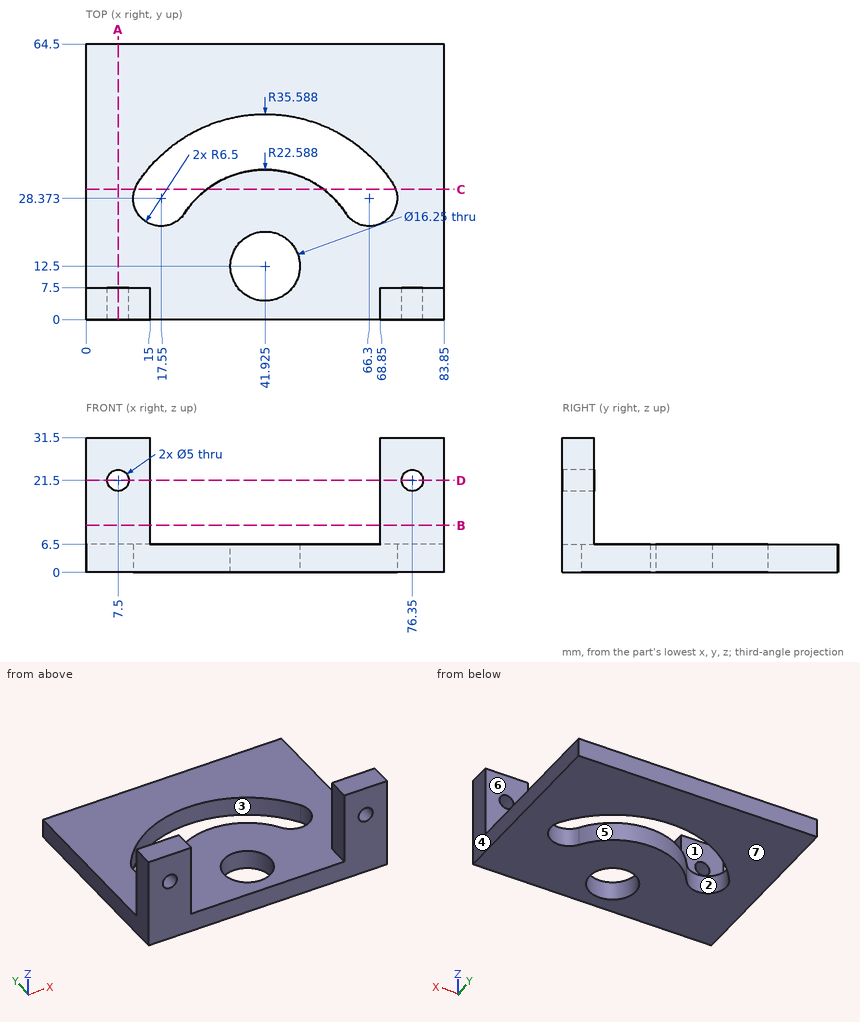
Source: three-view drawing plus pictorial views. Frame: mm from the lowest corner of the part. A direction names the side the tool comes from. Give positions to 0.01 mm unless a question says otherwise; leave off trailing zeros. Order: outer loops, then holes, each group sorted by start corner. A loop starts at its lowest first (then second) coordinate and runs counter-clockwise, first axis right, second up. Notation, with made-up numbers: (-15, 54.5) -> (30, 54.5) arc R24 ccw to (30, 86.5) -> close; hole circle Ø10 at (-4.75, 21). An arc over 180 degrees is marked (long way). Put each result on its own line as item: value.
Q1. Material intervals for L1, parallel to X at y = 4, z = 21; L2, parallel to Y at x = 21, z = 1.5 (1 decimal); L3, parallel to Z at x = 65, y = 46, sorted ascending.
Here are the results:
L1: x = 0 to 5.05, 9.95 to 15, 68.85 to 73.9, 78.8 to 83.85
L2: y = 0 to 22.9, 41.3 to 64.5
L3: z = 0 to 6.5
Q2. Section C-C, the plane y = 30.5. Return loops of the section in (x, z), then the cut area to 3 significant figures.
Here are the results:
outline: (0, 0) -> (11.41, 0) -> (11.41, 6.5) -> (0, 6.5) -> close; (28.28, 0) -> (55.57, 0) -> (55.57, 6.5) -> (28.28, 6.5) -> close; (72.44, 0) -> (83.85, 0) -> (83.85, 6.5) -> (72.44, 6.5) -> close
area: 326 mm^2
Q3. Reachability of the marked faces 5, 6 and 7 from +Z, -Z, +X, -X, +Y, -Y: full face, straight path, thin tool, end or side. Return the list, or none.
Here are the results:
face 5: +Z, -Z
face 6: +Z, +X, -X, +Y
face 7: -Z, +X, -X, +Y, -Y
Q4. Pin query (flat end, axial travel): pin 1 (12 mm diameter, centred on x = 75.5, z = 16.5, fed in from +Y); pin 2 (2 mm diameter, centred on x = 22, y = 55, fed in from +Z). Return the tip coordinate at first contact, or that it passes through.
Here are the results:
pin 1: stops at y = 7.5
pin 2: stops at z = 6.5
Q5. Draft query along X for the marked faces 1, 2, 3 and 4. Return one class per face: released by +X, released by -X, zero draft, split by the parting line, or undercut.
Here are the results:
face 1: zero draft
face 2: undercut
face 3: undercut
face 4: released by +X
Q6. Section B-B, the plane z = 11. Return loops of the section in (x, y).
Here are the results:
outline: (0, 0) -> (15, 0) -> (15, 7.5) -> (0, 7.5) -> close; (68.85, 0) -> (83.85, 0) -> (83.85, 7.5) -> (68.85, 7.5) -> close
Q7. Section D-D, the plane z = 21.5. Return loops of the section in (x, y).
Here are the results:
outline: (0, 0) -> (5, 0) -> (5, 7.5) -> (0, 7.5) -> close; (10, 0) -> (15, 0) -> (15, 7.5) -> (10, 7.5) -> close; (68.85, 0) -> (73.85, 0) -> (73.85, 7.5) -> (68.85, 7.5) -> close; (78.85, 0) -> (83.85, 0) -> (83.85, 7.5) -> (78.85, 7.5) -> close
Q8. Section A-A, the plane x = 7.5. Return loops of the section in (y, z).
Here are the results:
outline: (0, 0) -> (64.5, 0) -> (64.5, 6.5) -> (7.5, 6.5) -> (7.5, 19) -> (0, 19) -> close; (0, 24) -> (7.5, 24) -> (7.5, 31.5) -> (0, 31.5) -> close
